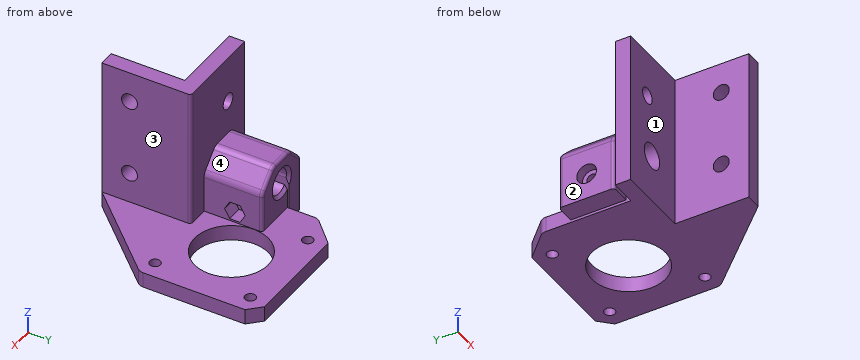
from build123d import *

# Parameters (mm, degrees)
SKETCH_R        = 12
SKETCH_R_2      = 1.75
PAD_DEPTH       = 5
PAD001_DEPTH    = 45
PAD002_DEPTH    = 19
POCKET_DEPTH    = 1
SKETCH004_R     = 4.15
POCKET001_DEPTH = 48.001
SKETCH005_R     = 2.6
POCKET002_DEPTH = 42.301
SKETCH006_R     = 2.6
POCKET003_DEPTH = 5
SKETCH008_R     = 1.75
POCKET004_DEPTH = 21.901
POCKET005_DEPTH = 5
SKETCH010_R     = 3.2
POCKET006_DEPTH = 3
SKETCH011_W     = 1
SKETCH011_H     = 10
POCKET007_DEPTH = 18.99
FILLET_R        = 3
FILLET001_R     = 1
CHAMFER_SIZE    = 1


with BuildPart() as part:
    # Sketch → Pad (new body)
    with BuildSketch(Plane.XY):
        Polygon((0, 0), (-24, 0), (-24, 5), (-15.5, 5), (-15.5, 33.95), (-7.15, 42.3), (27.15, 42.3), (31.15, 38.3), (31.15, 4), (5, -24), (0, -24), align=None)
        with Locations((10, 21.15)):
            Circle(SKETCH_R, mode=Mode.SUBTRACT)
        with Locations((-5.5, 36.65)):
            Circle(SKETCH_R_2, mode=Mode.SUBTRACT)
        with Locations((25.5, 36.65)):
            Circle(SKETCH_R_2, mode=Mode.SUBTRACT)
        with Locations((25.5, 5.65)):
            Circle(SKETCH_R_2, mode=Mode.SUBTRACT)
    extrude(amount=PAD_DEPTH)

    # Sketch001 (on Face17 of Pad) → Pad001 (join)
    with BuildSketch(Plane.XY.offset(5)):
        Polygon((0, 0), (-24, 0), (-24, 5), (5, 5), (5, -24), (0, -24), align=None)
    extrude(amount=PAD001_DEPTH)

    # Sketch002 (on Face19 of Pad001) → Pad002 (join)
    with BuildSketch(Plane(origin=(0, 5, 0), x_dir=(-1, 0, 0), z_dir=(0, 1, 0))):
        Polygon((22.9, 0), (22.9, 18), (16.9, 24), (8.1, 24), (2.1, 18), (2.1, 5), (16.5, 5), (16.5, 0), align=None)
    extrude(amount=PAD002_DEPTH)

    # Sketch003 (on Face25 of Pad002) → Pocket (cut)
    with BuildSketch(Plane(origin=(0, 5, 0), x_dir=(-1, 0, 0), z_dir=(0, 1, 0))):
        Polygon((15.5, 0), (15.5, 18), (19.2, 21.7), (22.9, 18), (22.9, 0), align=None)
    extrude(amount=POCKET_DEPTH, mode=Mode.SUBTRACT)

    # Sketch004 (on Face35 of Pocket) → Pocket001 (cut, through all)
    with BuildSketch(Plane(origin=(0, 24, 0), x_dir=(-1, 0, 0), z_dir=(0, 1, 0))):
        with Locations((12.5, 15.5)):
            Circle(SKETCH004_R)
    extrude(amount=-POCKET001_DEPTH, mode=Mode.SUBTRACT)

    # Sketch005 (on Face4 of Pocket001) → Pocket002 (cut, through all)
    with BuildSketch(Plane.XZ):
        with Locations((-15, 35)):
            Circle(SKETCH005_R)
    extrude(amount=-POCKET002_DEPTH, mode=Mode.SUBTRACT)

    # Sketch006 (on Face7 of Pocket002) → Pocket003 (cut)
    with BuildSketch(Plane(origin=(0, 0, 0), x_dir=(0, -1, 0), z_dir=(-1, 0, 0))):
        with Locations((15, 40)):
            Circle(SKETCH006_R)
        with Locations((15, 15)):
            Circle(SKETCH006_R)
    extrude(amount=-POCKET003_DEPTH, mode=Mode.SUBTRACT)

    # Sketch008 (on Face39 of Pocket003) → Pocket004 (cut, through all)
    with BuildSketch(Plane.YZ.offset(-2.1)):
        with Locations((15, 8.5)):
            Circle(SKETCH008_R)
    extrude(amount=-POCKET004_DEPTH, mode=Mode.SUBTRACT)

    # Sketch009 (on Face39 of Pocket004) → Pocket005 (cut)
    with BuildSketch(Plane.YZ.offset(-2.1)):
        Polygon((16.674316, 5.6), (18.348632, 8.5), (16.674316, 11.4), (13.325684, 11.4), (11.651368, 8.5), (13.325684, 5.6), align=None)
    extrude(amount=-POCKET005_DEPTH, mode=Mode.SUBTRACT)

    # Sketch010 (on Face42 of Pocket005) → Pocket006 (cut)
    with BuildSketch(Plane(origin=(-22.9, 0, 0), x_dir=(0, -1, 0), z_dir=(-1, 0, 0))):
        with Locations((-15, 8.5)):
            Circle(SKETCH010_R)
    extrude(amount=-POCKET006_DEPTH, mode=Mode.SUBTRACT)

    # Sketch011 (on Face35 of Pocket006) → Pocket007 (cut)
    with BuildSketch(Plane(origin=(0, 24, 0), x_dir=(-1, 0, 0), z_dir=(0, 1, 0))):
        with Locations((16, 10)):
            Rectangle(SKETCH011_W, SKETCH011_H)
    extrude(amount=-POCKET007_DEPTH, mode=Mode.SUBTRACT)

    # Fillet
    fillet_edges = [part.edges().sort_by_distance(p)[0] for p in [
        (31.15, 4, 2.5),
        (-15.5, 33.95, 2.5),
        (-2.1, 14.5, 18),
        (-8.1, 14.5, 24),
        (-16.9, 14.5, 24),
        (-22.9, 15, 18),
    ]]
    fillet(fillet_edges, radius=FILLET_R)

    # Fillet001
    fillet001_edges = [part.edges().sort_by_distance(p)[0] for p in [
        (5, 5, 27.5),
        (-2.1, 24, 10.87868),
        (-19.2, 5.5, 21.7),
        (-20.61066, 6, 20.28934),
    ]]
    fillet(fillet001_edges, radius=FILLET001_R)

    # Chamfer
    chamfer_edges = [part.edges().sort_by_distance(p)[0] for p in [
        (-8.648215, 24, 17.044749),
    ]]
    chamfer(chamfer_edges, length=CHAMFER_SIZE)


solid = part.part
The listing builds one solid part. Answer for the finished solid, in the listing's coordinates (mm). Face numbers are marked on the shaded views. A direction names the side the tool comes from. Give positions to 0.01 mm unless a question says otherwise; leave off trailing zeros. Order: outer loops, then holes, each group sorted by start corner. A loop starts at its lowest first (then second) coordinate and runs counter-clockwise, first axis right, second up. Notation, with made-up numbers: (45, -1.5) - (86, -1.5) arc R22 cw to (86, 18.5) - close; hole circle Ø10 at (13, -26). An arc over 180 degrees is marked (long way). Answer as CSV lines item,"result".
Q1. A cutting plane is placed at C-C, the plane x = 19. Determine the outline of the cut face in (y, z), and give its area (3 significant figures).
Answer key:
outline,"(-9.01, 0) - (13.21, 0) - (13.21, 5) - (-9.01, 5) - close; (29.09, 0) - (42.3, 0) - (42.3, 5) - (29.09, 5) - close"
area,"177 mm^2"
Q2. Each of these flat-tipped pins is pushed along its axis until it touches: pin 1 Ø6 at (y, z) = (15, 9) entering from +X; pin 2 Ø4 at (y, z) = (-9.5, 13) entering from +X; pin 3 Ø14.5 at (x, y) = (10, 21.15) entering from -Z; pin 4 Ø19 at (y, z) = (-11.5, 24) entering from -X. Where does it stop, or does it pass through?
Answer key:
pin 1,"stops at x = -2.1"
pin 2,"stops at x = 5"
pin 3,"passes through"
pin 4,"stops at x = 0"
Q3. Which of the six approach directions +Z, -Z, +X, -X, +Y, -Y give full straight-line access (tool end or side, diameter ignored) to the marked faces 1, 2, 3 and 4?
Answer key:
face 1,"+Z, -Z, -X, -Y"
face 2,"+Z, -Z, -X, +Y"
face 3,"+Z, +X, +Y, -Y"
face 4,"+Z, +X, +Y"
Q4. A cutting plane is placed at A-A, the plane y = 21.15. Determine the outline of the cut face in (x, z).
Answer key:
outline,"(-22.9, 0) - (-16.5, 0) - (-16.5, 14.39) arc R4.15 cw (long way) to (-15.5, 12.63) - (-15.5, 0) - (-2, 0) - (-2, 5) - (-2.1, 5) - (-2.1, 16.76) arc R3 ccw to (-2.98, 18.88) - (-7.22, 23.12) arc R3 ccw to (-9.34, 24) - (-15.66, 24) arc R3 ccw to (-17.78, 23.12) - (-22.02, 18.88) arc R3 ccw to (-22.9, 16.76) - close; (22, 0) - (31.15, 0) - (31.15, 5) - (22, 5) - close"
Q5. A cutting plane is placed at D-D, the plane x = 25.5. Determine the outline of the cut face in (y, z).
Answer key:
outline,"(-2.05, 0) - (3.9, 0) - (3.9, 5) - (-2.05, 5) - close; (7.4, 0) - (34.9, 0) - (34.9, 5) - (7.4, 5) - close; (38.4, 0) - (42.3, 0) - (42.3, 5) - (38.4, 5) - close"
Q6. Straight lines are drawn through the part: L1, parallel to X at y = 17, z = 4; L2, parallel to Z at x = 1.55, y = -15; L3, parallel to Y at x = 25, z = 2. For each, find the intervals that lie inside material, in ascending order.
Answer key:
L1,"x = -22.9 to -16.5, -15.5 to -1.26, 21.26 to 31.15"
L2,"z = 0 to 12.4, 17.6 to 37.4, 42.6 to 50"
L3,"y = -2.59 to 3.97, 7.33 to 34.97, 38.33 to 42.3"
Q7. A cutting plane is placed at B-B, the plane z = 34. Determine the outline of the cut face in (x, y), and give its area (3 significant figures).
Answer key:
outline,"(-24, 0) - (-17.4, 0) - (-17.4, 5) - (-24, 5) - close; (-12.6, 0) - (0, 0) - (0, -24) - (5, -24) - (5, 4) arc R1 ccw to (4, 5) - (-12.6, 5) - close"
area,"241 mm^2"
